CAD build for the part. Positions are in the model's coordinates, mm. Face numbers are marked on the shaded views. Coordinates: 2 decimals unless noted, no trailing zeros. Order: outer loops, then holes, each group sorted by start corner. A loop starts at its lowest first (then second) coordinate and runs counter-clockwise, first axis right, second up. Notation, with made-up numbers: M -31.5,59 L -7.5,59 A18 ccw -7.5,75 Z; hole C 23,10.25 d1. An arc over 180 degrees is marked long. Write item = value, one per line.
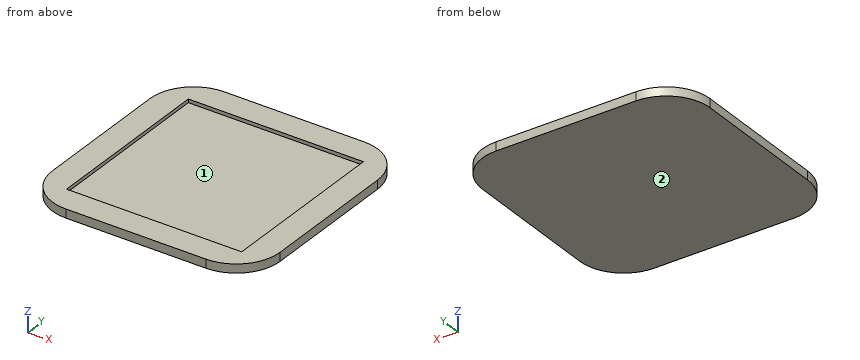
from build123d import *

# Parameters (mm, degrees)
F0_W     = 22
F0_H     = 22
F1_DEPTH = 0.6
F2_W     = 20
F2_H     = 20
F3_DEPTH = 1


with BuildPart() as f1:
    # F0 (on Top) → F1 (new body)
    with BuildSketch(Plane.XY):
        Rectangle(F0_W, F0_H)
    extrude(amount=F1_DEPTH)

    # F2 (on Top) → F3 (join)
    with BuildSketch(Plane.XY):
        with BuildLine():
            ThreePointArc((13, 8), (11.535534, 11.535534), (8, 13))
            Line((8, 13), (-8, 13))
            ThreePointArc((-8, 13), (-11.535534, 11.535534), (-13, 8))
            Line((-13, 8), (-13, -8))
            ThreePointArc((-13, -8), (-11.535534, -11.535534), (-8, -13))
            Line((-8, -13), (8, -13))
            ThreePointArc((8, -13), (11.535534, -11.535534), (13, -8))
            Line((13, -8), (13, 8))
        make_face()
        Rectangle(F2_W, F2_H, mode=Mode.SUBTRACT)
    extrude(amount=F3_DEPTH)


solid = f1.part
(1) Slice it at D-D, the plane y = -11. Write the cut outline in (x, z), then the cut area to 3 significant figures.
Evaluation:
outline = M -12,0 L 12,0 L 12,1 L -12,1 Z
area = 24.0 mm²
(2) Pin check, flat tip, straight feed: pin 1 Ø10 at (x, y) = (-2.5, 2.5) entering from +Z. Stop position of the tip, or through.
Evaluation:
pin_1 = 0.6
(3) Slice it at A-A, the plane z = 0.85. Write the cut outline in (x, y), then the cut area to 3 significant figures.
Evaluation:
outline = M -13,-8 A5 ccw -8,-13 L 8,-13 A5 ccw 13,-8 L 13,8 A5 ccw 8,13 L -8,13 A5 ccw -13,8 Z; hole M -10,-10 L 10,-10 L 10,10 L -10,10 Z
area = 255 mm²
(4) Wall check: line 1 (X direction, y = 3, z = 0.75); line 2 (Y direction, x = 8.25, z = 0.25). Give the ranges that are in metal, low to high. Write a range as from..to.
Evaluation:
line_1 = -13..-10, 10..13
line_2 = -12.99..12.99
(5) Slice it at B-B, the plane y = -3.5. Write the cut outline in (x, z).
Evaluation:
outline = M -13,0 L 13,0 L 13,1 L 10,1 L 10,0.6 L -10,0.6 L -10,1 L -13,1 Z
(6) Pull direction X, two halves, no side cores. Call the marked faces 1 and 2: +X half, -X half, draft (parallel to the pull), parting line (faces both ways), or undercut.
Evaluation:
face_1 = undercut
face_2 = draft
